Can you work these out from the model? Positions are in its coordinate system, mm. A direction names the side the tool comes from. Round coordinates to 2 decimals unless told otherwise and drop trailing zeros. Order: outer loops, then holes, each group sorted by start corner. A loop starts at its lowest first (then second) coordinate and runs counter-clockwise, first axis right, second up. Notation, with made-up numbers: (11, 46.25) - (27, 46.25) arc R26 cw to (27, 83.25) - close; hole circle Ø8 at (67, 17.25). An arc over 180 degrees is marked (long way). Write item = value, one per line.
from build123d import *

# Parameters (mm, degrees)
SKETCH1_R           = 1.5
BOSS_EXTRUDE1_DEPTH = 2
SKETCH2_R           = 1
SKETCH2_R_2         = 1.5
CUT_EXTRUDE1_DEPTH  = 2
CIRPATTERN1_COUNT   = 4


with BuildPart() as part:
    # Sketch1 → Boss-Extrude1 (new body)
    with BuildSketch(Plane(origin=(0, 0, 0), x_dir=(0, 0, -1), z_dir=(1, 0, 0))):
        with BuildLine():
            Line((0, 15), (-100, 15))
            Line((-100, 15), (-100, 7.5))
            Line((-100, 7.5), (-98, 7.5))
            Line((-98, 7.5), (-98, -7.5))
            Line((-98, -7.5), (-100, -7.5))
            Line((-100, -7.5), (-100, -15))
            Line((-100, -15), (-70.810782002, -15))
            Line((-70.810782002, -15), (-68.551280878, -15))
            Line((-68.551280878, -15), (0, -15))
            ThreePointArc((0, -15), (15, 0), (0, 15))
        make_face()
        Circle(SKETCH1_R, mode=Mode.SUBTRACT)
        Polygon((-91.077825525, 10), (-75.487484581, 10), (-91.077825525, -5.590340945), align=None, mode=Mode.SUBTRACT)
        Polygon((-86.66816647, -10), (-73.439167119, -10), (-71.179665994, -10), (-71.077825525, -10), (-71.077825525, 5.590340945), align=None, mode=Mode.SUBTRACT)
        Polygon((-47.487484581, -10), (-63.077825525, -10), (-63.077825525, 5.590340945), align=None, mode=Mode.SUBTRACT)
        Polygon((-43.077825525, -5.590340945), (-58.66816647, 10), (-43.077825525, 10), align=None, mode=Mode.SUBTRACT)
        Polygon((-35.077825525, 10), (-35.077825525, -5.590340945), (-19.487484581, 10), align=None, mode=Mode.SUBTRACT)
        Polygon((-15.077825525, 5.590340945), (-15.077825525, -10), (-30.66816647, -10), align=None, mode=Mode.SUBTRACT)
    extrude(amount=BOSS_EXTRUDE1_DEPTH)

    # Sketch2 → Cut-Extrude1 (cut)
    with BuildSketch(Plane.ZY):
        with Locations((6.5, 0)):
            Circle(SKETCH2_R)
        with Locations((66.885344311, 1.095113855)):
            Circle(SKETCH2_R_2)
        with Locations((66.822152611, -7.327248895)):
            Circle(SKETCH2_R_2)
    cut_extrude1 = extrude(amount=-CUT_EXTRUDE1_DEPTH, mode=Mode.SUBTRACT)

    # CirPattern1: Cut-Extrude1 ×4 about axis
    cirpattern1_axis = Axis((0, 0, 0), (1, 0, 0))
    for i in range(1, CIRPATTERN1_COUNT):
        add(cut_extrude1.rotate(cirpattern1_axis, i * 360 / CIRPATTERN1_COUNT), mode=Mode.SUBTRACT)


solid = part.part
(1) On a 3-axis mill with a long thin cutter (end or side, diameter ignored), from which of +Z, -Z, +X, -X, +Y, -Y can I reach the whole of each face in a straight line? I mean faces 1 (the face through (1, 0, 98)), 2 (the face through (1, 15, 49)), 3 (the face through (1, -2, 63.078)). Say none if no direction works.
Computed:
face_1 = +Z, +X, -X
face_2 = +Z, -Z, +X, -X, +Y
face_3 = +X, -X
(2) If I drill on line 1 (Y direction, x = 0.8, z = 50); line 2 (Z direction, x = 1.15, y = -8.25); line 3 (Z direction, x = 0.85, y = -6.5), over which ranges is the centre line in solid material (lowest first)? Write a range as from..to.
Computed:
line_1 = -15..-10, -7.49..1.33, 10..15
line_2 = -12.53..15.08, 28.92..49.24, 63.08..65.64, 68..71.08, 84.92..100
line_3 = -13.52..-1, 1..15.08, 27.17..50.99, 63.08..65.57, 68.07..71.08, 83.17..98
(3) If we section it at A-A (z = 6.5): Write out the boundary of the cut face in (x, y), plus the area to 3 significant figures.
Computed:
outline = (0, -15) - (2, -15) - (2, -1) - (0, -1) - close; (0, 1) - (2, 1) - (2, 15) - (0, 15) - close
area = 56.0 mm^2
(4) If we section it at B-B (y = 4): Write out the boundary of the cut face in (x, z), plus the area to 3 significant figures.
Computed:
outline = (0, -14.46) - (2, -14.46) - (2, 15.08) - (0, 15.08) - close; (0, 16.67) - (2, 16.67) - (2, 25.49) - (0, 25.49) - close; (0, 35.08) - (2, 35.08) - (2, 43.08) - (0, 43.08) - close; (0, 52.67) - (2, 52.67) - (2, 61.49) - (0, 61.49) - close; (0, 63.08) - (2, 63.08) - (2, 71.08) - (0, 71.08) - close; (0, 72.67) - (2, 72.67) - (2, 81.49) - (0, 81.49) - close; (0, 91.08) - (2, 91.08) - (2, 98) - (0, 98) - close
area = 158 mm^2
(5) Thinking about a two-plate mould opening in Z: for faces 4 (the face through (2, -6, 43)), 5 (the face through (1, 11, 100)), 6 (the face through (0.99, -2.31, 22.98)), which applies, +Z half, -Z half, draft (parallel to the pull), parting line (faces both ways), or undercut?
Computed:
face_4 = draft
face_5 = +Z half
face_6 = undercut
(6) Will this pin go through, and if not, where does the flat tip stop? P1, Ø1, axis at x = 1, y = 4.5, coming from the -Z side.
Computed:
P1 = -14.46
(7) If we section it at C-C (z = 81): Write out the boundary of the cut face in (x, y), plus the area to 3 significant figures.
Computed:
outline = (0, -15) - (2, -15) - (2, -10) - (0, -10) - close; (0, -4.33) - (2, -4.33) - (2, 4.49) - (0, 4.49) - close; (0, 10) - (2, 10) - (2, 15) - (0, 15) - close
area = 37.6 mm^2
(8) If we section it at D-D (x = 1.3): State how many separate pieces and enclosed holes the cut face has, plus the area to 3 significant figures.
Computed:
separate_pieces = 1
enclosed_holes = 13
area = 2,560 mm^2
